Geometry check sheet. Reference: the model listing, model coordinates, mm. A direction names the side the tool comes from. Give positions to 0.01 mm unless a question says otherwise; leave off trailing zeros. Loops run counter-clockwise (first coordinate to the right, second up) from the corner with the lowest first, then second, coordinate; pieces in that order, holes last. Notation, with made-up numbers: (75, 2) -> (88, 2) arc R13 ccw to (88, 10) -> close; hole circle Ø10 at (3.5, 39). An arc over 180 degrees is marked (long way). Answer in a Markdown table with one row per item. Add a question column.
```python
from build123d import *

# Parameters (mm, degrees)
SKETCH_1_R          = 2.75
EXTRUDE_1_DEPTH     = 3
FILLET_1_R          = 0.5
CUT_EXTRUDE_1_DEPTH = 2
SKETCH_3_R          = 1.5
EXTRUDE_2_DEPTH     = 16
CHAMFER_1_SIZE      = 0.2
FILLET_2_R          = 0.2


with BuildPart() as part:
    # 草图1 → 凸台-拉伸1 (new body)
    with BuildSketch(Plane.XY):
        Circle(SKETCH_1_R)
    extrude(amount=EXTRUDE_1_DEPTH)

    # 圆角1
    fillet_1_edges = [part.edges().sort_by_distance(p)[0] for p in [
        (-2.75, 0, 3),
    ]]
    fillet(fillet_1_edges, radius=FILLET_1_R)

    # 草图2 → 切除-拉伸1 (cut)
    with BuildSketch(Plane.XY.offset(3)):
        Polygon((1.558845727, 0), (0.779422863, 1.35), (-0.779422863, 1.35), (-1.558845727, 0), (-0.779422863, -1.35), (0.779422863, -1.35), align=None)
    extrude(amount=-CUT_EXTRUDE_1_DEPTH, mode=Mode.SUBTRACT)

    # 草图3 → 凸台-拉伸2 (add)
    with BuildSketch(Plane(origin=(0, 0, 0), x_dir=(-1, 0, 0), z_dir=(0, 0, -1))):
        Circle(SKETCH_3_R)
    extrude(amount=EXTRUDE_2_DEPTH)

    # 倒角1
    chamfer_1_edges = [part.edges().sort_by_distance(p)[0] for p in [
        (1.5, 0, -16),
    ]]
    chamfer(chamfer_1_edges, length=CHAMFER_1_SIZE)

    # 圆角2
    fillet_2_edges = [part.edges().sort_by_distance(p)[0] for p in [
        (-2.75, 0, 0),
    ]]
    fillet(fillet_2_edges, radius=FILLET_2_R)


solid = part.part
```
1. Release check for a two-part mould opening along Y. For faces 1 (the face through (1.5, -0.5, 3)), 2 (the face through (1.5, 0.07, -7.79)), 3 (the face through (-1.164, 0.684, 2.014)) record: released by +Y, released by -Y, zero draft, split by the parting line, or undercut.
2. Access from +Z, -Z, +X, -X, +Y, -Y to the whole of each face (thin tool, end or side, straight path). Record for faces 4 (the face through (1.164, -0.684, 2.014)), 5 (the face through (-0.596, -2.685, 1.334)), 6 (the face through (0, -2, 0)).
3. Sectioned sample at A-A (x = 0). Enter the section's corners in (y, z).
4. Material ranges on L1, parallel to X at y = 0.75, z = -2.75; L2, parallel to X at y = 0.4, z = 2; L3, parallel to Y at x = 0, z = -9, recorded low to high. Write a range as from..to.
5. Sectioned sample at C-C (z = -2.5). Enter the section's corners in (x, y).
6. Gauge pin test, flat ends, axial feed: pin 1 Ø3 at (y, z) = (0, -3) entering from -X; pin 2 Ø2 at (y, z) = (-1.5, -4) entering from -X; pin 3 Ø2 at (x, y) = (0, 0) entering from +Z. Record the tip position at first contact, or that the pin passes through.
7. Sectioned sample at B-B (z = 0.5). Enter the section's corners in (x, y), plus the area to 3 significant figures.
Response:
| question | item | result |
|---|---|---|
| 1 | face 1 | zero draft |
| 1 | face 2 | split by the parting line |
| 1 | face 3 | undercut |
| 2 | face 4 | +Z |
| 2 | face 5 | +Z, -Z |
| 2 | face 6 | -Z |
| 3 | outline | (-2.75, 0.2) arc R0.2 ccw to (-2.55, 0) -> (-1.5, 0) -> (-1.5, -15.8) -> (-1.3, -16) -> (1.3, -16) -> (1.5, -15.8) -> (1.5, 0) -> (2.55, 0) arc R0.2 ccw to (2.75, 0.2) -> (2.75, 2.5) arc R0.5 ccw to (2.25, 3) -> (1.35, 3) -> (1.35, 1) -> (-1.35, 1) -> (-1.35, 3) -> (-2.25, 3) arc R0.5 ccw to (-2.75, 2.5) -> close |
| 4 | L1 | x = -1.3..1.3 |
| 4 | L2 | x = -2.72..-1.33, 1.33..2.72 |
| 4 | L3 | y = -1.5..1.5 |
| 5 | outline | circle Ø3 at (0, 0) |
| 6 | pin 1 | stops at x = -1.5 |
| 6 | pin 2 | stops at x = -1.41 |
| 6 | pin 3 | stops at z = 1 |
| 7 | outline | circle Ø5.5 at (0, 0) |
| 7 | area | 23.8 mm2 |
